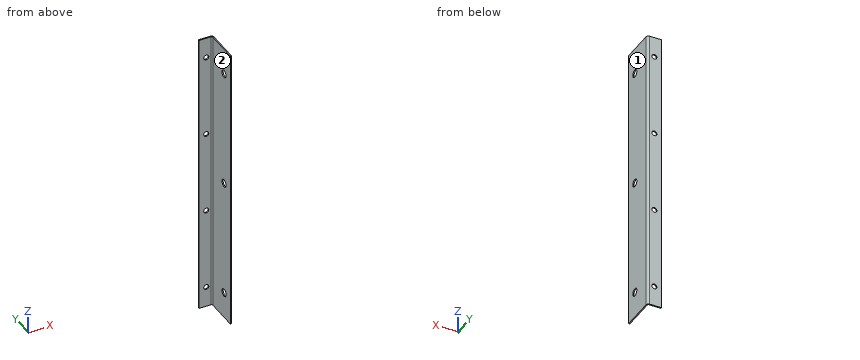
from build123d import *

# Parameters (mm, degrees)
EXTRUDE_1_DEPTH     = 245
SKETCH_2_R          = 2.15
CUT_EXTRUDE_1_DEPTH = 245
SKETCH_3_R          = 3.25
CUT_EXTRUDE_2_DEPTH = 245


with BuildPart() as part:
    # Эскиз1 → Вытянуть1 (new body)
    with BuildSketch(Plane.XY):
        with BuildLine():
            Line((-1, -2), (-1, -30))
            Line((-1, -30), (0, -30))
            Line((0, -30), (0, -2))
            ThreePointArc((0, -2), (-0.585786438, -0.585786438), (-2, 0))
            Line((-2, 0), (-12, 0))
            Line((-12, 0), (-12, -1))
            Line((-12, -1), (-2, -1))
            ThreePointArc((-2, -1), (-1.292893219, -1.292893219), (-1, -2))
        make_face()
    extrude(amount=EXTRUDE_1_DEPTH)

    # Эскиз2 → Вырез-Вытянуть1 (cut)
    with BuildSketch(Plane(origin=(0, 0, 0), x_dir=(1, 0, 0), z_dir=(0, 1, 0))):
        with Locations(Location((-6, -17.5, 0), (0, 0, 180))):
            Circle(SKETCH_2_R)
        with Locations(Location((-6, -87.5, 0), (0, 0, 180))):
            Circle(SKETCH_2_R)
        with Locations(Location((-6, -157.5, 0), (0, 0, 180))):
            Circle(SKETCH_2_R)
        with Locations(Location((-6, -227.5, 0), (0, 0, 180))):
            Circle(SKETCH_2_R)
    extrude(amount=-CUT_EXTRUDE_1_DEPTH, mode=Mode.SUBTRACT)

    # Эскиз3 → Вырез-Вытянуть2 (cut)
    with BuildSketch(Plane(origin=(0, 0, 0), x_dir=(0, 0, -1), z_dir=(1, 0, 0))):
        with Locations(Location((-122.5, -20, 0), (0, 0, 90))):
            Circle(SKETCH_3_R)
        with Locations(Location((-22.5, -20, 0), (0, 0, 90))):
            Circle(SKETCH_3_R)
        with Locations((-222.5, -20)):
            Circle(SKETCH_3_R)
    extrude(amount=-CUT_EXTRUDE_2_DEPTH, mode=Mode.SUBTRACT)


solid = part.part
Input: part model. Units: mm. Frame: model coordinates. Face numbers are marked on the shaded views. A direction names the side the tool comes from. Round coordinates to 2 decimals unless told otherwise and drop trailing zeros. Order: outer loops, then holes, each group sorted by start corner. A loop starts at its lowest first (then second) coordinate and runs counter-clockwise, first axis right, second up.
1. Cut plane C-C, the plane z = 22.5. Output: boundary loops of the cut face in (x, y).
The answers:
outline: (-12, -1) - (-2, -1) arc R1 cw to (-1, -2) - (-1, -16.75) - (0, -16.75) - (0, -2) arc R2 ccw to (-2, 0) - (-12, 0) - close; (-1, -30) - (0, -30) - (0, -23.25) - (-1, -23.25) - close
2. Material intervals for line 1 (Z direction, x = -6, y = -0.3); line 2 (X direction, y = -8.5, z = 180), sorted ascending.
The answers:
line 1: z = 0 to 15.35, 19.65 to 85.35, 89.65 to 155.35, 159.65 to 225.35, 229.65 to 245
line 2: x = -1 to 0
3. Pin query (flat end, axial travel): P1, Ø7, axis at x = -6, z = 227.5, coming from the -Y side; P2, Ø8.5, axis at y = -20, z = 122.5, coming from the -X side. Return the tip coordinate at first contact, or that it passes through.
The answers:
P1: stops at y = -1
P2: stops at x = -1
4. Cut plane B-B, the plane y = -20. Output: boundary loops of the cut face in (x, z), then the cut area to 4 significant figures.
The answers:
outline: (-1, 0) - (0, 0) - (0, 19.25) - (-1, 19.25) - close; (-1, 25.75) - (0, 25.75) - (0, 119.25) - (-1, 119.25) - close; (-1, 125.75) - (0, 125.75) - (0, 219.25) - (-1, 219.25) - close; (-1, 225.75) - (0, 225.75) - (0, 245) - (-1, 245) - close
area: 225.5 mm2
5. Cut plane D-D, the plane z = 145. Output: boundary loops of the cut face in (x, y).
The answers:
outline: (-12, -1) - (-2, -1) arc R1 cw to (-1, -2) - (-1, -30) - (0, -30) - (0, -2) arc R2 ccw to (-2, 0) - (-12, 0) - close
6. Cut plane A-A, the plane x = -6. Output: boundary loops of the cut face in (y, z).
The answers:
outline: (-1, 0) - (0, 0) - (0, 15.35) - (-1, 15.35) - close; (-1, 19.65) - (0, 19.65) - (0, 85.35) - (-1, 85.35) - close; (-1, 89.65) - (0, 89.65) - (0, 155.35) - (-1, 155.35) - close; (-1, 159.65) - (0, 159.65) - (0, 225.35) - (-1, 225.35) - close; (-1, 229.65) - (0, 229.65) - (0, 245) - (-1, 245) - close
7. Set-up query: the marked faces 1 and 2. Return all of +Z, -Z, +X, -X, +Y, -Y with unobstructed straight access to the full face (end or side cutting, diameter ignored); none if empty.
The answers:
face 1: +Z, -Z, +X, +Y, -Y
face 2: +Z, -Z, -X, -Y
